Autodesk Inventor part; units mm, degrees
ref_plane "YZ Plane" through (0, 0, 0) normal (1, 0, 0) x (0, 1, 0)
ref_plane "XZ Plane" through (0, 0, 0) normal (0, 1, 0) x (-1, 0, 0)
ref_plane "XY Plane" through (0, 0, 0) normal (0, 0, 1) x (1, 0, 0)
sketch "Sketch1" plane through (0, 0, 0) normal (0, 1, 0) x (-1, 0, 0)
  line L0 (330.2, 153.9875) -> (-330.2, 153.9875)
  line L1 (-330.2, 153.9875) -> (-330.2, -153.9875)
  line L2 (-330.2, -153.9875) -> (330.2, -153.9875)
  line L3 (330.2, -153.9875) -> (330.2, 153.9875)
  line L4 (330.2, 153.9875) -> (-330.2, -153.9875) construction
  line L5 (-330.2, 153.9875) -> (330.2, -153.9875) construction
  point P0 (0, 0)
  dimension "d0" = 660.4
  dimension "d1" = 307.975
extrude "Extrusion1" add sketch "Sketch1" along normal blind 374.65
sketch "Sketch4" plane through (330.2, 0, 153.9875) normal (1, 0, 0) x (0, 0, -1)
  line L0 (96.8375, 161.925) -> (211.1375, 161.925)
  line L1 (211.1375, 161.925) -> (211.1375, 238.125)
  line L2 (211.1375, 238.125) -> (96.8375, 238.125)
  line L3 (96.8375, 238.125) -> (96.8375, 161.925)
  point P0 (153.9875, 0)
  point P1 (153.9875, 161.925)
  dimension "d11" = 114.3
  dimension "d12" = 161.925
  dimension "d13" = 76.2
extrude "Extrusion4" add sketch "Sketch4" along normal blind 12.7
mirror "Mirror1" about plane through (0, 0, 0) normal (1, 0, 0) of "Extrusion4"
sketch "Sketch6" plane through (-330.2, 0, 153.9875) normal (0, 0, 1) x (1, 0, 0)
  line L0 (0, 374.65) -> (660.4, 374.65)
  line L1 (0, 374.65) -> (0, 9.525)
  line L2 (0, 9.525) -> (660.4, 9.525)
  line L3 (660.4, 9.525) -> (660.4, 374.65)
  point P0 (330.2, 0)
  dimension "d22" = 9.525
extrude "Extrusion6" add sketch "Sketch6" along normal blind 1.5875
fillet "Fillet1" radius 50.8 1 edges at (0, 374.65, 155.575)
properties part number "Blue tool box" material "Steel"
Build history of the part. All positions in model axes, mm. A direction names the side the tool comes from. Round coordinates to 2 decimals unless told otherwise and drop trailing zeros. Write each loop counter-clockwise with the first axis right and the second up, starting at its lowest first coordinate (ties: lowest second). Pieces come first, ordered by that corner, then holes. Notation, with made-up numbers: (81.25, -5) - (133.25, -5) arc R31 ccw to (133.25, 31) - close; hole circle Ø5 at (82.25, 40). An arc over 180 degrees is marked (long way). Write each question's results on one line, items separated by ' | '. Start each with the question number.
Item 1: Which spindle directions (+Z, -Z, +X, -X, +Y, -Y) get a long thin tool onto all of the face, cutting with end or side? Do faces 1 (the face through (-336, 199, 57.15)), 2 (the face through (336, 161.925, 1)), 3 (the face through (-336, 201, -57.15)). Say none if no direction does.
Item 2: Wall check: L1, parallel to X at y = 209, z = -83.5; L2, parallel to Z at x = 161.5, y = 341.5; L3, parallel to Z at x = -57, y = 348. Give the ranges that are in metal, low to high. Write a range as [from, to].
Item 3: Drop flat-ended pins along their axis: P1, Ø5, axis at y = 233, z = -106.5, coming from the -X side; P2, Ø5, axis at x = -138, z = -8, coming from the -Y side; P3, Ø3, axis at x = -51.5, y = 2.5, coming from the +Z side; P4, Ø14, axis at x = 338, z = -1, coming from the -Y side (3 decimals). Give the stop position or say it passes through.
Item 4: Saw through at C-C (y = 263). Write the cut outline in (x, z) (1 decimal).
Item 5: Saw through at B-B (z = -132). Write the cut outline in (x, y), and give its area (3 significant figures).
Results are:
1) face 1: +Z, -X, +Y, -Y | face 2: +Z, -Z, +X, -Y | face 3: -Z, -X, +Y, -Y
2) L1: x = [-330.2, 330.2] | L2: z = [-153.99, 152.41] | L3: z = [-153.99, 149.47]
3) P1: stops at x = -330.2 | P2: stops at y = 0 | P3: stops at z = 153.99 | P4: stops at y = 161.925
4) outline: (-330.2, -154) - (330.2, -154) - (330.2, 155.6) - (-330.2, 155.6) - close
5) outline: (-330.2, 0) - (330.2, 0) - (330.2, 374.65) - (-330.2, 374.65) - close | area: 247,000 mm²
